from build123d import *

# Parameters (mm, degrees)
SKETCH_1_W          = 120
SKETCH_1_H          = 90
EXTRUDE_1_DEPTH     = 5
SKETCH_5_W          = 120
SKETCH_5_H          = 10
CUT_EXTRUDE_3_DEPTH = 10
SKETCH_10_W         = 5
SKETCH_10_H         = 5.002587902
EXTRUDE_3_DEPTH     = 15
SKETCH_12_W         = 5
SKETCH_12_H         = 5.002587902
EXTRUDE_4_DEPTH     = 15
SKETCH_14_W         = 3
SKETCH_14_H         = 15.404940373
EXTRUDE_5_DEPTH     = 5
SKETCH_16_W         = 5
SKETCH_16_H         = 29.952587902
CUT_EXTRUDE_5_DEPTH = 10
SKETCH_17_W         = 5
SKETCH_17_H         = 29.952587902
CUT_EXTRUDE_6_DEPTH = 10
SKETCH_18_W         = 10
SKETCH_18_H         = 4
SKETCH_18_W_2       = 7
SKETCH_18_H_2       = 20
CUT_EXTRUDE_7_DEPTH = 10
SKETCH_19_W         = 1.5
SKETCH_19_H         = 3
EXTRUDE_6_DEPTH     = 5
SKETCH_20_R         = 5.5
SKETCH_20_R_2       = 1.5
CUT_EXTRUDE_8_DEPTH = 10


with BuildPart() as part:
    # 草图1 → 凸台-拉伸1 (new body)
    with BuildSketch(Plane.XY):
        Rectangle(SKETCH_1_W, SKETCH_1_H)
    extrude(amount=EXTRUDE_1_DEPTH)

    # 草图5 → 切除-拉伸3 (cut)
    with BuildSketch(Plane(origin=(0, 0, 0), x_dir=(-1, 0, 0), z_dir=(0, 0, -1))):
        with Locations((0, -40)):
            Rectangle(SKETCH_5_W, SKETCH_5_H)
    extrude(amount=-CUT_EXTRUDE_3_DEPTH, mode=Mode.SUBTRACT)

    # 草图10 → 凸台-拉伸3 (add)
    with BuildSketch(Plane(origin=(60, 0, 0), x_dir=(0, 0, -1), z_dir=(1, 0, 0))):
        with Locations((-2.5, -2.501293951)):
            Rectangle(SKETCH_10_W, SKETCH_10_H)
    extrude(amount=EXTRUDE_3_DEPTH)

    # 草图12 → 凸台-拉伸4 (add)
    with BuildSketch(Plane.ZY.offset(60)):
        with Locations((2.5, -2.501293951)):
            Rectangle(SKETCH_12_W, SKETCH_12_H)
    extrude(amount=EXTRUDE_4_DEPTH)

    # 草图14 → 凸台-拉伸5 (add, through all)
    with BuildSketch(Plane(origin=(0, 0, 0), x_dir=(-1, 0, 0), z_dir=(0, 0, -1))):
        with Locations((-61.5, 7.702470187)):
            Rectangle(SKETCH_14_W, SKETCH_14_H)
        with Locations((61.5, 7.702470187)):
            Rectangle(SKETCH_14_W, SKETCH_14_H)
    extrude(amount=-EXTRUDE_5_DEPTH)

    # 草图16 → 切除-拉伸5 (cut)
    with BuildSketch(Plane(origin=(0, 0, 0), x_dir=(-1, 0, 0), z_dir=(0, 0, -1))):
        with Locations((60.5, 30.023706049)):
            Rectangle(SKETCH_16_W, SKETCH_16_H)
        with Locations((-60.5, 30.023706049)):
            Rectangle(SKETCH_16_W, SKETCH_16_H)
    extrude(amount=-CUT_EXTRUDE_5_DEPTH, mode=Mode.SUBTRACT)

    # 草图17 → 切除-拉伸6 (cut)
    with BuildSketch(Plane(origin=(0, 0, 0), x_dir=(-1, 0, 0), z_dir=(0, 0, -1))):
        with Locations((-55.5, 30.023706049)):
            Rectangle(SKETCH_17_W, SKETCH_17_H)
        with Locations((55.5, 30.023706049)):
            Rectangle(SKETCH_17_W, SKETCH_17_H)
    extrude(amount=-CUT_EXTRUDE_6_DEPTH, mode=Mode.SUBTRACT)

    # 草图18 → 切除-拉伸7 (cut)
    with BuildSketch(Plane(origin=(0, 0, 0), x_dir=(-1, 0, 0), z_dir=(0, 0, -1))):
        with Locations((-58, 13.047412098)):
            Rectangle(SKETCH_18_W, SKETCH_18_H)
        with Locations((-56.5, -25)):
            Rectangle(SKETCH_18_W_2, SKETCH_18_H_2)
        with Locations((56.5, -25)):
            Rectangle(SKETCH_18_W_2, SKETCH_18_H_2)
        with Locations((58, 13.047412098)):
            Rectangle(SKETCH_18_W, SKETCH_18_H)
    extrude(amount=-CUT_EXTRUDE_7_DEPTH, mode=Mode.SUBTRACT)

    # 草图19 → 凸台-拉伸6 (add, through all)
    with BuildSketch(Plane(origin=(0, 0, 0), x_dir=(-1, 0, 0), z_dir=(0, 0, -1))):
        with Locations((-63.75, 1.5)):
            Rectangle(SKETCH_19_W, SKETCH_19_H)
        with Locations((63.75, 1.5)):
            Rectangle(SKETCH_19_W, SKETCH_19_H)
    extrude(amount=-EXTRUDE_6_DEPTH)

    # 草图20 → 切除-拉伸8 (cut)
    with BuildSketch(Plane(origin=(0, 0, 0), x_dir=(-1, 0, 0), z_dir=(0, 0, -1))):
        with Locations((0, 5)):
            Circle(SKETCH_20_R)
        with Locations((6, 11)):
            Circle(SKETCH_20_R_2)
        with Locations((6, -1)):
            Circle(SKETCH_20_R_2)
        with Locations((-6, -1)):
            Circle(SKETCH_20_R_2)
        with Locations((-6, 11)):
            Circle(SKETCH_20_R_2)
    extrude(amount=-CUT_EXTRUDE_8_DEPTH, mode=Mode.SUBTRACT)


solid = part.part
The listing builds one solid part. Answer for the finished solid, in the listing's coordinates (mm). A direction names the side the tool comes from. Give positions to 0.01 mm unless a question says otherwise; leave off trailing zeros. Write each loop counter-clockwise with the first axis right and the second up, starting at its lowest first coordinate (ties: lowest second). Pieces come first, ordered by that corner, then holes. Notation, with made-up numbers: (23.25, 34) -> (70.25, 34) arc R25 cw to (70.25, 63) -> close; hole circle Ø3 at (24.25, 11). An arc over 180 degrees is marked (long way). Use a Markdown table: item, result.
(1) Section D-D, the plane x = -56.5 is taken. Determine the outline of the cut face in (y, z), then the cut area to 3 significant figures.
Return value:
| item | result |
|---|---|
| outline | (-15, 0) -> (11.05, 0) -> (11.05, 5) -> (-15, 5) -> close |
| area | 130 mm2 |
(2) Section A-A, the plane x = 0 is taken. Determine the outline of the cut face in (y, z).
Return value:
| item | result |
|---|---|
| outline | (-35, 0) -> (-0.5, 0) -> (-0.5, 5) -> (-35, 5) -> close; (10.5, 0) -> (45, 0) -> (45, 5) -> (10.5, 5) -> close |
(3) Section B-B, the plane y = 5 is taken. Determine the outline of the cut face in (x, z).
Return value:
| item | result |
|---|---|
| outline | (-63, 0) -> (-5.5, 0) -> (-5.5, 5) -> (-63, 5) -> close; (5.5, 0) -> (63, 0) -> (63, 5) -> (5.5, 5) -> close |
(4) Section C-C, the plane z = 2.55 is taken. Give the number of separate pieces and of enclosed holes in the cut face, then the cut area to 3 significant figures.
Return value:
| item | result |
|---|---|
| separate pieces | 1 |
| enclosed holes | 5 |
| area | 8,950 mm2 |
(5) Flat-ended cylindrical pins translate along their axes: P1, Ø1.5, axis at y = 1.5, z = 2.5, coming from the -X side; P2, Ø2.5, axis at y = 7.5, z = 3.5, coming from the -X side; P3, Ø1.5, axis at y = 2, z = 1.5, coming from the +X side; P4, Ø3.5, axis at x = -6, y = -1, coming from the +Z side. Find the tip coordinate at first contact, or state that the pin passes through.
Return value:
| item | result |
|---|---|
| P1 | x = -64.5 |
| P2 | x = -63 |
| P3 | x = 64.5 |
| P4 | z = 5 |
(6) For faces 5 (the flat face through (67, -5.003, 3)), 6 (the flat face through (58, 11.047, 2)), 7 (the flat face through (-56, -15, 2)), 8 (the flat face through (-63, 7, 2)), determine the directions among +Z, -Z, +X, -X, +Y, -Y from which every point of the face is accessible in a straight line to the end or side of a thin tool.
Return value:
| item | result |
|---|---|
| face 5 | +Z, -Z, +X, -Y |
| face 6 | +Z, -Z, +X, +Y |
| face 7 | +Z, -Z, -X, -Y |
| face 8 | +Z, -Z, -X, +Y |
(7) Find the intervals of material crossed by probe 1 along Y at (x, z) = (6, 1.5); probe 2 along Y at (x, z) = (0, 1.8); probe 3 along X at (y, z) = (-29, 2.8), in increasing order. Write a range as from..to.
Return value:
| item | result |
|---|---|
| probe 1 | -35..-2.5, 0.5..9.5, 12.5..45 |
| probe 2 | -35..-0.5, 10.5..45 |
| probe 3 | -53..53 |
(8) Determine the mould class of faces 1 (the flat face through (-67, -5.003, 2)), 2 (the flat face through (1, -3, 0)), 3 (the cylindrical face through (-4.8, 10.1, 2.5)), 4 (the cylindrical face through (7.2, -1.9, 2.5)) for opening direction Y: released by +Y, released by -Y, zero draft, split by the parting line, or undercut.
Return value:
| item | result |
|---|---|
| face 1 | released by -Y |
| face 2 | zero draft |
| face 3 | undercut |
| face 4 | undercut |
